Could you check a few things on this model? Use its own coordinates, in mm. A direction names the side the tool comes from. Give positions to 0.01 mm unless a question says otherwise; leave off trailing zeros. Loops run counter-clockwise (first coordinate to the right, second up) from the corner with the lowest first, then second, coordinate; pieces in that order, holes last. Notation, with made-up numbers: M 64.5,46.5 L 91.5,46.5 A27 cw 91.5,66.5 Z; hole C 56,82.5 d8. An arc over 180 degrees is marked long. Use a Markdown table: item, result. Add a question column.
1) Suppose I cut it at C-C on y = 23.5. List the corners of the cut face in (x, z) for me.
2) We'd pull the mould along Y, two halves only. Please class faces 4 (the cylindrical face through (78.86, -16.848, -0.424)), 5 (the cylindrical face through (68.75, -13.29, 2.2)), 6 (the flat face through (69, 3, -14)): +Y half, -Y half, draft (parallel to the pull), parting line (faces both ways), or undercut.
3) Will these pins go through, and if not, where does the flat tip stop? pin 1 Ø11 at (y, z) = (12.5, -3) entering from +X; pin 2 Ø3 at (y, z) = (1, 3.5) entering from -X.
4) Which directions (+Z, -Z, +X, -X, +Y, -Y) give clear straight access to the entire face, cutting with the end or side of a thin tool? Please do faces 1 (the flat face through (-75.5, 3, 6)), 2 (the cylindrical face through (68.75, 19.82, 2.07)), 3 (the cylindrical face through (-75.25, 19.69, 2.2)).
5) Suppose I cut it at A-A on y = -6. List the corners of the cut face in (x, z) for me.
6) If I drill on line 1 along X through (y, z) = (-11, -5.5); line 2 along X through (y, z) = (19, 4.5), over which ranges is the centre line in solid material (lowest first)? Write a range as [from, to].
7) Suppose I cut it at B-B on z = -7.5. List the corners of the cut face in (x, y) for me, and give its area (3 significant figures).
```python
from build123d import *

# Parameters (mm, degrees)
SKETCH1_W           = 144.5
SKETCH1_H           = 50.4
BOSS_EXTRUDE1_DEPTH = 22.26
CUT_EXTRUDE1_DEPTH  = 0.5
CUT_EXTRUDE2_START  = -0.5
CUT_EXTRUDE2_DEPTH  = 0.5
SKETCH5_R           = 2
BOSS_EXTRUDE2_DEPTH = 20
SKETCH6_R           = 2
BOSS_EXTRUDE3_DEPTH = 20


with BuildPart() as part:
    # Sketch1 → Boss-Extrude1 (new body)
    with BuildSketch(Plane(origin=(0, 0, -15), x_dir=(-1, 0, 0), z_dir=(0, 0, -1))):
        with Locations((3.25, 3.2)):
            Rectangle(SKETCH1_W, SKETCH1_H)
    extrude(amount=-BOSS_EXTRUDE1_DEPTH)

    # Sketch2 → Cut-Extrude1 (cut)
    with BuildSketch(Plane(origin=(69, 0, 0), x_dir=(0, 0, -1), z_dir=(1, 0, 0))):
        with BuildLine():
            Line((-4.4775, 14.1), (-4.4775, -7.7))
            ThreePointArc((-4.4775, -7.7), (-2.134354249, -13.356854249), (3.5225, -15.7))
            Line((3.5225, -15.7), (4.2175, -15.7))
            ThreePointArc((4.2175, -15.7), (9.874354249, -13.356854249), (12.2175, -7.7))
            Line((12.2175, -7.7), (12.2175, 14.1))
            ThreePointArc((12.2175, 14.1), (9.874354249, 19.756854249), (4.2175, 22.1))
            Line((4.2175, 22.1), (3.5225, 22.1))
            ThreePointArc((3.5225, 22.1), (-2.134354249, 19.756854249), (-4.4775, 14.1))
        make_face()
    extrude(amount=-CUT_EXTRUDE1_DEPTH, mode=Mode.SUBTRACT)

    # Sketch3 → Cut-Extrude2 (cut)
    with BuildSketch(Plane.ZY.offset(75.5).offset(CUT_EXTRUDE2_START)):
        with BuildLine():
            Line((-3.5225, 22.1), (-4.2175, 22.1))
            ThreePointArc((-4.2175, 22.1), (-9.874354249, 19.756854249), (-12.2175, 14.1))
            Line((-12.2175, 14.1), (-12.2175, -7.7))
            ThreePointArc((-12.2175, -7.7), (-9.874354249, -13.356854249), (-4.2175, -15.7))
            Line((-4.2175, -15.7), (-3.5225, -15.7))
            ThreePointArc((-3.5225, -15.7), (2.134354249, -13.356854249), (4.4775, -7.7))
            Line((4.4775, -7.7), (4.4775, 14.1))
            ThreePointArc((4.4775, 14.1), (2.134354249, 19.756854249), (-3.5225, 22.1))
        make_face()
    extrude(amount=CUT_EXTRUDE2_DEPTH, mode=Mode.SUBTRACT)

    # Sketch5 → Boss-Extrude2 (add)
    with BuildSketch(Plane(origin=(69, 0, 0), x_dir=(0, 0, -1), z_dir=(1, 0, 0))):
        with Locations((-0.651385293, -18.534553966)):
            Circle(SKETCH5_R)
    extrude(amount=BOSS_EXTRUDE2_DEPTH)

    # Sketch6 → Boss-Extrude3 (add)
    with BuildSketch(Plane(origin=(69, 0, 0), x_dir=(0, 0, -1), z_dir=(1, 0, 0))):
        with Locations((-4.774830425, -18.459565293)):
            Circle(SKETCH6_R)
    extrude(amount=BOSS_EXTRUDE3_DEPTH)


solid = part.part
```
Answer block:
| question | item | result |
|---|---|---|
| 1 | outline | M -75.5,-15 L 69,-15 L 69,7.26 L -75.5,7.26 Z |
| 2 | face 4 | parting line |
| 2 | face 5 | undercut |
| 2 | face 6 | draft |
| 3 | pin 1 | stops at x = 68.5 |
| 3 | pin 2 | stops at x = -75.5 |
| 4 | face 1 | +Z, -Z, -X, +Y, -Y |
| 4 | face 2 | +X |
| 4 | face 3 | -X |
| 5 | outline | M -75.5,-15 L 69,-15 L 69,-12.22 L 68.5,-12.22 L 68.5,4.48 L 69,4.48 L 69,7.26 L -75.5,7.26 L -75.5,4.48 L -75,4.48 L -75,-12.22 L -75.5,-12.22 Z |
| 6 | line 1 | x = [-75, 68.5] |
| 6 | line 2 | x = [-75.5, 69] |
| 7 | outline | M -75.5,-22 L 69,-22 L 69,-15 L 68.5,-15 L 68.5,21.4 L 69,21.4 L 69,28.4 L -75.5,28.4 L -75.5,21.4 L -75,21.4 L -75,-15 L -75.5,-15 Z |
| 7 | area | 7,250 mm^2 |
